Verification items for this drawing (mm, ordinates from the low corner). Coordinates: 2 decimals unless noted, no trailing zeros. Order: outer loops, then holes, each group sorted by start corner. A loop starts at its lowest first (then second) coordinate and runs counter-clockwise, first axis right, second up. Notation, with made-up numbers: (34.25, -22) - (40.25, -22) arc R28 ccw to (40.25, 6) - close; hole circle Ø8 at (86.5, 54.5). An arc over 180 degrees is marked (long way). One line per question, with ' | ' between items. Start each with the question number.
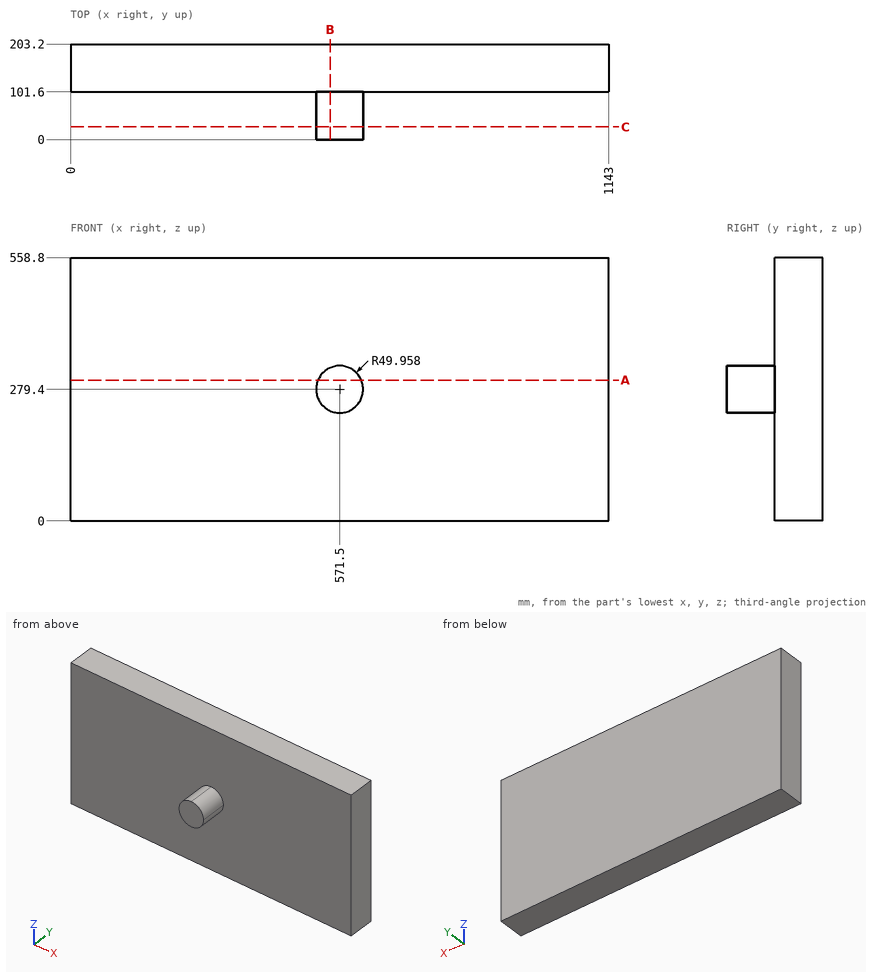
Item 1: Section check C-C (y = 27). Record the cut outline in (x, z).
Item 2: Gauge pin test, flat end, axial feed: pin 1 (10 mm diameter, centred on x = 726.5, z = 191.5, fed in from -Y). Record the tip position at first contact, or that the pin passes through.
Item 3: Section check B-B (x = 551.5). Record the cut outline in (y, z), then the cut area to 3 significant figures.
Item 4: Section check A-A (z = 299). Record the cut outline in (x, y), then the cut area to 3 significant figures.
Item 5: Thickness scan on probe 1 along Y at (x, z) = (471.5, 202.5); probe 2 along Z at (x, y) = (591.5, 15); probe 3 along X at (y, z) = (15.5, 295). Record the ranges inside material, lowest first. Write a range as from..to.
Completed:
1) outline: (521.54, 279.4) arc R49.96 ccw to (571.5, 229.44) arc R49.96 ccw to (621.46, 279.4) arc R49.96 ccw to (571.5, 329.36) arc R49.96 ccw to start
2) pin 1: stops at y = 101.6
3) outline: (0, 233.62) - (101.6, 233.62) - (101.6, 0) - (203.2, 0) - (203.2, 558.8) - (101.6, 558.8) - (101.6, 325.18) - (0, 325.18) - close | area: 66,100 mm^2
4) outline: (0, 101.6) - (525.55, 101.6) - (525.55, 0) - (617.45, 0) - (617.45, 101.6) - (1143, 101.6) - (1143, 203.2) - (0, 203.2) - close | area: 125,000 mm^2
5) probe 1: y = 101.6..203.2 | probe 2: z = 233.62..325.18 | probe 3: x = 524.04..618.96
